The model under review builds one solid part; all positions refer to its coordinate system, in mm. Face numbers are marked on the shaded views. A direction names the side the tool comes from. Give positions to 0.01 mm unless a question says otherwise; leave off trailing zeros. Loops run counter-clockwise (first coordinate to the right, second up) from the corner with the lowest first, then second, coordinate; pieces in that order, holes last. Notation, with made-up numbers: M 88.25,-6 L 135.25,-6 A22 cw 135.25,9 Z; hole C 52,18 d4. An arc over 180 degrees is marked long. Return JSON: item names as keys, results as strings.
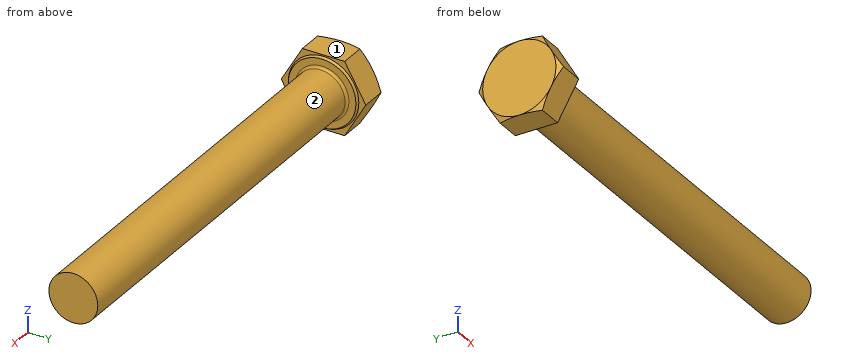
```python
from build123d import *

# Parameters (mm, degrees)
EXTRUDE_382_DEPTH = 7.5
FILLET_1274_R     = 0.6


with BuildPart() as part:
    # 草图1 → Extrude 382 (new body)
    with BuildSketch(Plane(origin=(0, 0, 0), x_dir=(0, 0, -1), z_dir=(1, 0, 0))):
        Polygon((9, 5.196152423), (9, -5.196152423), (0, -10.392304845), (-9, -5.196152423), (-9, 5.196152423), (0, 10.392304845), align=None)
    extrude(amount=EXTRUDE_382_DEPTH)

    # 草图2 → 凸台-旋转1 (revolve)
    with BuildSketch(Plane.XY):
        Polygon((0, 0), (107.5, 0), (107.5, 4.4845), (107.5, 6), (77.5, 6), (0, 6), align=None)
    revolve(axis=Axis((0, 0, 0), (1, 0, 0)))

    # 草图3 → 切除-旋转1 (revolve, cut)
    with BuildSketch(Plane.XY):
        Polygon((0, 9), (3.690598923, 15.392304845), (3.690598923, 20.392304845), (-10, 20.392304845), (-10, 9), align=None)
    revolve(axis=Axis((0, 0, 0), (1, 0, 0)), mode=Mode.SUBTRACT)

    # 草图4 → 切除-旋转3 (revolve, cut)
    with BuildSketch(Plane.XY):
        Polygon((7.5, 8.315), (6.9, 8.661410162), (6.9, 10.392304845), (7.5, 10.392304845), align=None)
    revolve(axis=Axis((0, 0, 0), (1, 0, 0)), mode=Mode.SUBTRACT)

    # Fillet 1274
    fillet_1274_edges = [part.edges().sort_by_distance(p)[0] for p in [
        (7.5, -6, 0),
    ]]
    fillet(fillet_1274_edges, radius=FILLET_1274_R)


solid = part.part
```
1) Consider section A-A on x = 75. Write out the cut boundary in (y, z).
From the geometry:
{"outline": "C 0,0 d12"}
2) Tool access review of the marked faces 1 and 2: name each direction out of +Z, -Z, +X, -X, +Y, -Y from which nothing blocks a thin tool from reaching the whole face with its end or side.
From the geometry:
{"face 1": "+Z, +X, -X, +Y, -Y", "face 2": "+X"}
3) Wall thickness on L1, parallel to Z at x = 79, y = -0.25; L2, parallel to X at y = -7.5, z = 0.25; L3, parallel to Z at x = 20, y = -3: over which ranges is each line inside the solid? List them lowest first. Write a range as from..to.
From the geometry:
{"L1": "-5.99..5.99", "L2": "0..7.5", "L3": "-5.2..5.2"}
4) Insertion check: pin 1 (1.5 mm diameter, centred on x = 60, y = 4, fed in from -Z); pin 2 (2 mm diameter, centred on x = 47.5, z = 5, fed in from -Y); pin 3 (3 mm diameter, centred on x = 52, z = 2.5, fed in from +Y). Each pin has a flat end and moves straight along its axis. Give the tip position at first contact, or say it passes through.
From the geometry:
{"pin 1": "z = -5.04", "pin 2": "y = -4.47", "pin 3": "y = 5.92"}
